The model under review builds one solid part; all positions refer to its coordinate system, in mm. A direction names the side the tool comes from. Round coordinates to 2 decimals unless told otherwise and drop trailing zeros. Write each loop counter-clockwise with the first axis right and the second up, starting at its lowest first coordinate (ties: lowest second). Pieces come first, ordered by that corner, then holes. Notation, with made-up numbers: (-35, 39.25) - (-10, 39.25) arc R22 ccw to (-10, 71.25) - close; hole circle Ø4 at (1, 24.5). An arc over 180 degrees is marked (long way). Use one line per item in the form item = value.
from build123d import *

# Parameters (mm, degrees)
SKETCH2_R          = 1.9939
CUT_EXTRUDE1_DEPTH = 29.792891484
SKETCH3_R          = 5.715
CUT_EXTRUDE2_DEPTH = 3.81


with BuildPart() as part:
    # Sketch1 → Revolve1 (revolve)
    with BuildSketch(Plane(origin=(0, 0, 0), x_dir=(0, 0, -1), z_dir=(1, 0, 0)), mode=Mode.PRIVATE) as revolve1_sk:
        Polygon((17.2847, 0), (7.1247, 0), (7.1247, 12.2555), (6.3627, 12.2555), (6.3627, 14.2875), (0, 14.2875), (0, 16.51), (7.6327, 16.51), (7.6327, 19.05), (10.1727, 19.05), (10.1727, 10.795), (17.2847, 10.795), align=None)
    revolve(revolve1_sk.sketch.rotate(Axis((0, 0, 32.351737074), (0, 0, -1)), 90), axis=Axis((0, 0, 32.351737074), (0, 0, -1)))

    # Sketch2 → Cut-Extrude1 (cut, through all)
    with BuildSketch(Plane.XY.offset(-7.1247)):
        Circle(SKETCH2_R)
    extrude(amount=-CUT_EXTRUDE1_DEPTH, mode=Mode.SUBTRACT)

    # Sketch3 → Cut-Extrude2 (cut)
    with BuildSketch(Plane.XY.offset(-7.1247)):
        Circle(SKETCH3_R)
    extrude(amount=-CUT_EXTRUDE2_DEPTH, mode=Mode.SUBTRACT)


solid = part.part
(1) Insertion check: P1, Ø2.5, axis at x = 0, y = 0, coming from the +Z side; P2, Ø5, axis at y = 1, z = -13, coming from the +X side (3 decimals); P3, Ø10, axis at x = -3, z = -9.5, coming from the -Y side; P4, Ø3, axis at x = 6.5, y = -7.5, coming from the +Z side. Each pin has a flat end and moves straight along its axis. Give the tip position at first contact, or say it passes through.
Geometry results:
P1 = through
P2 = 10.795
P3 = -19.05
P4 = -7.12
(2) The part is to be moulded in two halves that separate along Y. For faces 1 (the flat face through (-0.2, 2.2, -17.285)), 2 (the cylindrical face through (1.9, 0.6, -14.1)), 3 (the cylindrical face through (-4.13, 18.597, -8.92)), say which applies: +Y half, -Y half, draft (parallel to the pull), parting line (faces both ways), or undercut.
Geometry results:
face_1 = draft
face_2 = undercut
face_3 = parting line
(3) Add section C-C on y = -16. Write out the cut boundary in (x, z), then the cut area to 3 significant figures.
Geometry results:
outline = (-10.34, -10.17) - (10.34, -10.17) - (10.34, -7.63) - (4.07, -7.63) - (4.07, 0) - (-4.07, 0) - (-4.07, -7.63) - (-10.34, -7.63) - close
area = 115 mm2
(4) Add section D-D on z = -3.5. Write out the cut boundary in (x, y) (1 decimal), then the cut area to 3 significant figures.
Geometry results:
outline = circle Ø33 at (0, 0); hole circle Ø28.6 at (0, 0)
area = 215 mm2
(5) Machinability: for faces 4 (the cylindrical face through (-7.956, -7.296, -13.778)), 5 (the cylindrical face through (5.45, 1.72, -9)), 6 (the flat face through (5, -14, 0)), which of the approach directions +Z, -Z, +X, -X, +Y, -Y give a long, thin tool a straight path to every point of the face, cutting with its end or side? Answer none if there is none.
Geometry results:
face_4 = -Z
face_5 = +Z
face_6 = +Z, +X, -X, +Y, -Y
(6) To check wall thickness, follow L1, parallel to Y at x = 0, z = -1.75; L2, parallel to Y at x = 0, z = -12.25 (3 decimals); L3, parallel to X at y = 12.5, z = -7. State the ranges of each line that lie inside material, in increasing order.
Geometry results:
L1 = -16.51 to -14.29, 14.29 to 16.51
L2 = -10.795 to -1.994, 1.994 to 10.795
L3 = -10.79 to 10.79
